The listing builds one solid part. Answer for the finished solid, in the listing's coordinates (mm). A direction names the side the tool comes from. Coordinates: 2 decimals unless noted, no trailing zeros. Loops run counter-clockwise (first coordinate to the right, second up) from the corner with the lowest first, then second, coordinate; pieces in that order, holes last. Notation, with made-up numbers: M 54.5,-2.5 L 83.5,-2.5 A11 cw 83.5,5.5 Z; hole C 2,12.25 d1. An arc over 180 degrees is marked long. Answer as CSV lines item,"result". Start each with the question number.
```python
from build123d import *

# Parameters (mm, degrees)
BOSS_EXTRUDE1_DEPTH = 64
BOSS_EXTRUDE2_DEPTH = 5
SKETCH5_R           = 2.75
BOSS_EXTRUDE3_DEPTH = 8
SKETCH6_R           = 4.5
CUT_EXTRUDE1_DEPTH  = 5
SKETCH7_R           = 2.75
SKETCH7_R_2         = 5
CUT_EXTRUDE2_DEPTH  = 131.241540308
SKETCH8_R           = 4.5
CUT_EXTRUDE3_DEPTH  = 14
FILLET2_R           = 20


with BuildPart() as part:
    # Sketch3 → Boss-Extrude1 (new body)
    with BuildSketch(Plane.XY):
        with BuildLine():
            Line((0, 0), (50, 0))
            Line((50, 0), (50, 20))
            ThreePointArc((50, 20), (25, 15.993420768), (0, 20))
            Line((0, 20), (0, 0))
        make_face()
    extrude(amount=BOSS_EXTRUDE1_DEPTH)

    # Sketch4 → Boss-Extrude2 (add)
    with BuildSketch(Plane(origin=(0, 0, 0), x_dir=(-1, 0, 0), z_dir=(0, 0, -1))):
        with BuildLine():
            Line((-50, 0), (0, 0))
            Line((0, 0), (0, 25))
            ThreePointArc((0, 25), (-25, 20.726789434), (-50, 25))
            Line((-50, 25), (-50, 0))
        make_face()
    extrude(amount=BOSS_EXTRUDE2_DEPTH)

    # Sketch5 → Boss-Extrude3 (add)
    with BuildSketch(Plane.XY.offset(64)):
        with BuildLine():
            Line((0, 0), (50, 0))
            Line((50, 0), (50, 45.536190526))
            Line((50, 45.536190526), (69.276231493, 68.902511677))
            ThreePointArc((69.276231493, 68.902511677), (67.66630765, 80.565752686), (56.176914536, 77.993420768))
            ThreePointArc((56.176914536, 77.993420768), (54.575493633, 75.468066292), (52.77001177, 73.084329859))
            Line((52.77001177, 73.084329859), (31.171113727, 46.902511677))
            ThreePointArc((31.171113727, 46.902511677), (25, 43.993420768), (18.828886273, 46.902511677))
            Line((18.828886273, 46.902511677), (-2.77001177, 73.084329859))
            ThreePointArc((-2.77001177, 73.084329859), (-4.575493633, 75.468066292), (-6.176914536, 77.993420768))
            ThreePointArc((-6.176914536, 77.993420768), (-17.66630765, 80.565752686), (-19.276231493, 68.902511677))
            Line((-19.276231493, 68.902511677), (0, 45.536190526))
            Line((0, 45.536190526), (0, 0))
        make_face()
        with Locations((63.105117767, 73.993420768)):
            Circle(SKETCH5_R, mode=Mode.SUBTRACT)
        with Locations((-13.105117767, 73.993420768)):
            Circle(SKETCH5_R, mode=Mode.SUBTRACT)
    extrude(amount=BOSS_EXTRUDE3_DEPTH)

    # Sketch6 → Cut-Extrude1 (cut)
    with BuildSketch(Plane.XY.offset(72)):
        with Locations((-13.105117767, 73.993420768)):
            Circle(SKETCH6_R)
        with Locations((63.105117767, 73.993420768)):
            Circle(SKETCH6_R)
    extrude(amount=-CUT_EXTRUDE1_DEPTH, mode=Mode.SUBTRACT)

    # Sketch7 → Cut-Extrude2 (cut, through all)
    with BuildSketch(Plane.XZ):
        with Locations(Location((25, 44, 0), (0, 0, 270))):
            Circle(SKETCH7_R)
        with Locations(Location((36.412678196, 35.708203932, 0), (0, 0, 270))):
            Circle(SKETCH7_R)
        with Locations(Location((32.053423028, 22.291796068, 0), (0, 0, 270))):
            Circle(SKETCH7_R)
        with Locations(Location((17.946576972, 22.291796068, 0), (0, 0, 270))):
            Circle(SKETCH7_R)
        with Locations(Location((13.587321804, 35.708203932, 0), (0, 0, 270))):
            Circle(SKETCH7_R)
        with Locations(Location((25, 32, 0), (0, 0, 270))):
            Circle(SKETCH7_R_2)
    extrude(amount=-CUT_EXTRUDE2_DEPTH, mode=Mode.SUBTRACT)

    # Sketch8 → Cut-Extrude3 (cut)
    with BuildSketch(Plane(origin=(0, 20, 0), x_dir=(1, 0, 0), z_dir=(0, 1, 0))):
        with Locations(Location((25, -44, 0), (0, 0, 180))):
            Circle(SKETCH8_R)
        with Locations(Location((17.946576972, -22.291796068, 0), (0, 0, 180))):
            Circle(SKETCH8_R)
        with Locations(Location((32.053423028, -22.291796068, 0), (0, 0, 180))):
            Circle(SKETCH8_R)
        with Locations(Location((36.412678196, -35.708203932, 0), (0, 0, 180))):
            Circle(SKETCH8_R)
        with Locations(Location((13.587321804, -35.708203932, 0), (0, 0, 180))):
            Circle(SKETCH8_R)
    extrude(amount=-CUT_EXTRUDE3_DEPTH, mode=Mode.SUBTRACT)

    # Fillet2
    fillet2_edges = [part.edges().sort_by_distance(p)[0] for p in [
        (0, 45.536190526, 68),
        (50, 45.536190526, 68),
    ]]
    fillet(fillet2_edges, radius=FILLET2_R)


solid = part.part
```
Item 1: Section C-C on y = 14 is taken. Determine the outline of the cut face in (x, z).
Item 2: For faces 1 (the face through (8.18, 59.81, 67.94)), 2 (the face through (35.359, 2.958, 33.168)), 3 (the face through (40.91, 11.88, 35.91)), 4 (the face through (62.519, 78.455, 69.535)), 5 (the face through (24.643, 20.728, -2.465)), determine the directions among +Z, -Z, +X, -X, +Y, -Y from which every point of the face is accessible in a straight line to the end or side of a thin tool.
Item 3: Section B-B on x = 25 is taken. Determine the outline of the cut face in (y, z), then the cut area to 3 significant figures.
Item 4: Each of these flat-tipped pins is pushed along its axis until it touches: P1, Ø7, axis at x = 16, z = 24, coming from the +Y side; P2, Ø7, axis at x = 32.05, z = 22.29, coming from the +Y side; P3, Ø7, axis at x = 38.5, z = 37.5, coming from the +Y side; P4, Ø10, axis at x = -14, y = 73, coming from the +Z side. Where does it stop, or does it pass through?
Item 5: Consider line 1 (Z direction, x = 25, y = 9); line 2 (X direction, y = 10, z = 32); line 3 (Y direction, x = 20.5, z = 19). Determine where each line is inside the solid, lowest interval first.
Item 6: For a pull along Y with two mould halves and no side action, classify faces 6 (the face through (34, 6, 38)), 7 (the face through (63, 71, 67)), 8 (the face through (67.817, 80.458, 67.944)) as pulls with the +Y half, pulls with the -Y half, needs draft (parallel to the pull), parting line crosses it, or undercut.
Item 7: Section A-A on z = 44 is taken. Determine the outline of the cut face in (x, y).
Item 8: Section D-D on x = 64 is taken. Determine the outline of the cut face in (y, z), then the cut area to 3 significant figures.
Results are:
1,outline,"M 0,-5 L 50,-5 L 50,72 L 0,72 Z; hole C 13.59,35.71 d9; hole C 17.95,22.29 d9; hole C 25,32 d10; hole C 25,44 d9; hole C 32.05,22.29 d9; hole C 36.41,35.71 d9"
2,face 1,"+Z, -Z, +Y"
2,face 2,"+Y, -Y"
2,face 3,"+Y"
2,face 4,"+Z"
2,face 5,"-Z, +Y"
3,outline,"M 0,-5 L 20.73,-5 L 20.73,0 L 15.99,0 L 15.99,27 L 0,27 Z; M 0,37 L 15.99,37 L 15.99,39.5 L 6,39.5 L 6,41.25 L 0,41.25 Z; M 0,46.75 L 6,46.75 L 6,48.5 L 15.99,48.5 L 15.99,64 L 43.99,64 L 43.99,72 L 0,72 Z"
3,area,"1,200 mm²"
4,P1,"y = 16.98"
4,P2,"y = 6"
4,P3,"y = 17.82"
4,P4,"z = 72"
5,line 1,"-5 to 27, 37 to 39.5, 48.5 to 72"
5,line 2,"0 to 11.04, 16.14 to 20, 30 to 33.86, 38.96 to 50"
5,line 3,"0 to 6"
6,face 6,"pulls with the +Y half"
6,face 7,"undercut"
6,face 8,"parting line crosses it"
7,outline,"M 0,0 L 22.25,0 L 22.25,6 L 20.5,6 L 20.5,16.12 A80 cw 0,20 Z; M 27.75,0 L 50,0 L 50,20 A80 cw 29.5,16.12 L 29.5,6 L 27.75,6 Z"
8,outline,"M 62.51,64 L 71.39,64 L 71.39,67 L 69.58,67 L 69.58,72 L 62.51,72 Z; M 76.59,64 L 81.94,64 L 81.94,72 L 78.4,72 L 78.4,67 L 76.59,67 Z"
8,area,"95.8 mm²"
